from build123d import *

# Parameters (mm, degrees)
SKETCH1_R           = 6.35
SKETCH1_R_2         = 3.175
BOSS_EXTRUDE1_DEPTH = 5.08
SKETCH1_3_R         = 3.175
BOSS_EXTRUDE2_DEPTH = 49.53
BOSS_EXTRUDE3_START = -49.53
SKETCH1_4_R         = 16.51
SKETCH1_4_R_2       = 6.35
SKETCH1_4_R_3       = 3.175
BOSS_EXTRUDE3_DEPTH = 7.62


with BuildPart() as part:
    # Sketch1 → Boss-Extrude1 (new body)
    # profile 1 of 2: a face of its own
    with BuildSketch(Plane(origin=(0, 0, 0), x_dir=(1, 0, 0), z_dir=(0, 1, 0))):
        with Locations(Location((0, 0, 0), (0, 0, 270))):
            Circle(SKETCH1_R)
        Circle(SKETCH1_R_2, mode=Mode.SUBTRACT)
    # profile 2 of 2: a face of its own
    with BuildSketch(Plane(origin=(0, 0, 0), x_dir=(1, 0, 0), z_dir=(0, 1, 0))):
        Circle(SKETCH1_R_2)
    extrude(amount=BOSS_EXTRUDE1_DEPTH)

    # Sketch1<3> → Boss-Extrude2 (add)
    with BuildSketch(Plane(origin=(0, 0, 0), x_dir=(1, 0, 0), z_dir=(0, 1, 0))):
        with Locations(Location((0, 0, 0), (0, 0, 270))):
            Circle(SKETCH1_3_R)
    extrude(amount=-BOSS_EXTRUDE2_DEPTH)

    # Sketch1<4> → Boss-Extrude3 (add)
    # profile 1 of 3: a face of its own
    with BuildSketch(Plane(origin=(0, 0, 0), x_dir=(1, 0, 0), z_dir=(0, 1, 0)).offset(BOSS_EXTRUDE3_START)):
        with Locations(Location((0, 0, 0), (0, 0, 270))):
            Circle(SKETCH1_4_R)
        with Locations(Location((0, 0, 0), (0, 0, 270))):
            Circle(SKETCH1_4_R_2, mode=Mode.SUBTRACT)
    # profile 2 of 3: a face of its own
    with BuildSketch(Plane(origin=(0, 0, 0), x_dir=(1, 0, 0), z_dir=(0, 1, 0)).offset(BOSS_EXTRUDE3_START)):
        with Locations(Location((0, 0, 0), (0, 0, 270))):
            Circle(SKETCH1_4_R_2)
        with Locations(Location((0, 0, 0), (0, 0, 270))):
            Circle(SKETCH1_4_R_3, mode=Mode.SUBTRACT)
    # profile 3 of 3: a face of its own
    with BuildSketch(Plane(origin=(0, 0, 0), x_dir=(1, 0, 0), z_dir=(0, 1, 0)).offset(BOSS_EXTRUDE3_START)):
        with Locations(Location((0, 0, 0), (0, 0, 270))):
            Circle(SKETCH1_4_R_3)
    extrude(amount=-BOSS_EXTRUDE3_DEPTH)


solid = part.part
Model file for the job. Use its own axes, mm. A direction names the side the tool comes from. Round coordinates to 2 decimals unless told otherwise and drop trailing zeros. Loops run counter-clockwise (first coordinate to the right, second up) from the corner with the lowest first, then second, coordinate; pieces in that order, holes last.
1. Band-saw the part on A-A, the plane z = 0. List the corners of the cut face in (x, y) (3 decimals).
Check values:
outline: (-16.51, -57.15) - (16.51, -57.15) - (16.51, -49.53) - (3.175, -49.53) - (3.175, 0) - (6.35, 0) - (6.35, 5.08) - (-6.35, 5.08) - (-6.35, 0) - (-3.175, 0) - (-3.175, -49.53) - (-16.51, -49.53) - close
2. Wall check: probe 1 along Y at (x, z) = (-4, 0); probe 2 along Y at (x, z) = (8.5, 13); probe 3 along X at (y, z) = (-33, -2). Give the ranges that are in metal, low to high.
Check values:
probe 1: y = -57.15 to -49.53, 0 to 5.08
probe 2: y = -57.15 to -49.53
probe 3: x = -2.47 to 2.47
3. Drop flat-ended pins along their axis: P1, Ø5, axis at x = 7, y = -29.5, coming from the -Z side; P2, Ø12, axis at x = 2.5, y = -17.5, coming from the -Z side (3 decimals); P3, Ø6, axis at y = -16, z = -3.5, coming from the +X side. Give the stop position or say it passes through.
Check values:
P1: passes through
P2: stops at z = -3.175
P3: stops at x = 3.14
4. Band-saw the part on D-D, the plane y = -7. List the corners of the cut face in (x, z) (3 decimals).
Check values:
outline: circle Ø6.35 at (0, 0)
5. Band-saw the part on C-C, the plane x = 5.5. List the corners of the cut face in (y, z).
Check values:
outline: (-57.15, -15.57) - (-49.53, -15.57) - (-49.53, 15.57) - (-57.15, 15.57) - close; (0, -3.17) - (5.08, -3.17) - (5.08, 3.17) - (0, 3.17) - close
6. Mould opens along Y. For faces 4 (the flat face through (0, -57.15, 0)), 5 (the cylindrical face through (-10.05, -53.29, -13.1)), 6 (the cylindrical face through (-1.93, -24.42, -2.52)) say: +Y half, -Y half, draft (parallel to the pull), parting line (faces both ways), or undercut.
Check values:
face 4: -Y half
face 5: draft
face 6: undercut
7. Band-saw the part on B-B, the plane x = 0. List the corners of the cut face in (y, z) (3 decimals), and give its area (3 significant figures).
Check values:
outline: (-57.15, -16.51) - (-49.53, -16.51) - (-49.53, -3.175) - (0, -3.175) - (0, -6.35) - (5.08, -6.35) - (5.08, 6.35) - (0, 6.35) - (0, 3.175) - (-49.53, 3.175) - (-49.53, 16.51) - (-57.15, 16.51) - close
area: 631 mm2
8. Tool access for faces 1 (the flat face through (-2, 0, -3)), 2 (the cylindrical face through (-3.86, 2.5, -5.04)), 3 (the flat face through (0, 5.08, 0)): list every direction of +Z, -Z, +X, -X, +Y, -Y with a clear straight run to the whole face (end or side of a thin tool).
Check values:
face 1: none
face 2: +Y
face 3: +Z, -Z, +X, -X, +Y
